```python
from build123d import *

# Parameters (mm, degrees)
BOSS_EXTRUDE1_DEPTH  = 8
M3_CLEARANCE_HOLE1_D = 3.6
FILLET1_R            = 1
SKETCH5_W            = 4
SKETCH5_H            = 7
CUT_EXTRUDE1_DEPTH   = 4
FILLET2_R            = 1


with BuildPart() as part:
    # Sketch1 → Boss-Extrude1 (new body)
    with BuildSketch(Plane.XY):
        Polygon((-16.25, -7.5), (-11.5, -7.5), (-11.5, 0), (3.5, 0), (3.5, 4), (11.5, 4), (11.5, -7.5), (16.25, -7.5), (16.25, 7), (-16.25, 7), align=None)
    extrude(amount=BOSS_EXTRUDE1_DEPTH)

    # M3 Clearance Hole1 (through all)
    with Locations(Plane(origin=(0, 7, 0), x_dir=(1, 0, 0), z_dir=(0, 1, 0))):
        with Locations((13.75, -4), (-13.75, -4)):
            Hole(M3_CLEARANCE_HOLE1_D / 2)

    # Fillet1
    fillet1_edges = [part.edges().sort_by_distance(p)[0] for p in [
        (-16.25, -0.25, 8),
        (-16.25, -0.25, 0),
        (16.25, -0.25, 0),
        (16.25, -0.25, 8),
    ]]
    fillet(fillet1_edges, radius=FILLET1_R)

    # Sketch5 → Cut-Extrude1 (cut)
    with BuildSketch(Plane(origin=(0, 0, 0), x_dir=(-1, 0, 0), z_dir=(0, 0, -1))):
        with Locations((-9, 3.5)):
            Rectangle(SKETCH5_W, SKETCH5_H)
    extrude(amount=-CUT_EXTRUDE1_DEPTH, mode=Mode.SUBTRACT)

    # Fillet2
    fillet2_edges = [part.edges().sort_by_distance(p)[0] for p in [
        (11, 5.5, 4),
        (7, 5.5, 4),
    ]]
    fillet(fillet2_edges, radius=FILLET2_R)


solid = part.part
```
Check sheet for the modelled part. Datum: model origin and axes. Units: mm. A direction names the side the tool comes from. Give positions to 0.01 mm unless a question says otherwise; leave off trailing zeros. Order: outer loops, then holes, each group sorted by start corner. A loop starts at its lowest first (then second) coordinate and runs counter-clockwise, first axis right, second up. Notation, with made-up numbers: (84, -31) -> (135, -31) arc R15 ccw to (135, -12) -> close; hole circle Ø4 at (55.5, -19.5). An arc over 180 degrees is marked (long way). Use CSV: the item, a comma, the result in double quotes. Start each with the question number.
1) Go/stop test with flat-tipped pins: P1, Ø1, axis at x = 8.5, y = 5, coming from the -Z side; P2, Ø1.5, axis at x = -1.5, z = 4, coming from the -Y side. Record where each tip stops, or that it passes through.
2) Set-up check for faces 1 (the face through (-4, 0, 4)), 2 (the face through (14, -7.5, 2)), 3 (the face through (11, 5, 1)): record each of +Z, -Z, +X, -X, +Y, -Y from which the full face is reachable in a straight line by a thin tool's end or side.
3) Mould release check, pull along X, two halves, no side actions. Record for faces 4 (the face through (7.285, 5.521, 3.699)), 5 (the face through (16.25, 0, 4)), 6 (the face through (13, 0, 0)): released by +X, released by -X, zero draft, split by the parting line, or undercut.
4) Sectioned sample at D-D, the plane x = 13. Record the boundary of the cut face in (y, z), plus the area to 3 significant figures.
5) Material ranges on line 1 (X direction, y = -0.25, z = 4); line 2 (X direction, y = 3.5, z = 4); line 3 (Z direction, x = -13.75, y = 2.5), recorded low to high. Write a range as from..to.
6) Sectioned sample at C-C, the plane y = -5.5. Record the boundary of the cut face in (x, z).
7) Sectioned sample at A-A, the plane y = 0.75. Record the boundary of the cut face in (x, z).
8) Sectioned sample at B-B, the plane x = -13.75. Record the boundary of the cut face in (y, z), plus the area to 3 significant figures.
Recorded:
1,P1,"z = 4"
1,P2,"y = 0"
2,face 1,"+Z, -Z, -Y"
2,face 2,"+Z, -Z, +X, -X, -Y"
2,face 3,"-Z, +Y, -Y"
3,face 4,"undercut"
3,face 5,"released by +X"
3,face 6,"zero draft"
4,outline,"(-7.5, 0) -> (7, 0) -> (7, 2.36) -> (-7.5, 2.36) -> close; (-7.5, 5.64) -> (7, 5.64) -> (7, 8) -> (-7.5, 8) -> close"
4,area,"68.5 mm2"
5,line 1,"-16.25..-15.55, -11.95..-11.5, 11.5..11.95, 15.55..16.25"
5,line 2,"-16.25..-15.55, -11.95..3.5, 11.5..11.95, 15.55..16.25"
5,line 3,"0..2.2, 5.8..8"
6,outline,"(-16.25, 1) arc R1 ccw to (-15.25, 0) -> (-11.5, 0) -> (-11.5, 8) -> (-15.25, 8) arc R1 ccw to (-16.25, 7) -> close; (11.5, 0) -> (15.25, 0) arc R1 ccw to (16.25, 1) -> (16.25, 7) arc R1 ccw to (15.25, 8) -> (11.5, 8) -> close; hole circle Ø3.6 at (-13.75, 4); hole circle Ø3.6 at (13.75, 4)"
7,outline,"(-16.25, 1) arc R1 ccw to (-15.25, 0) -> (3.5, 0) -> (3.5, 8) -> (-15.25, 8) arc R1 ccw to (-16.25, 7) -> close; (11.5, 0) -> (15.25, 0) arc R1 ccw to (16.25, 1) -> (16.25, 7) arc R1 ccw to (15.25, 8) -> (11.5, 8) -> close; hole circle Ø3.6 at (-13.75, 4); hole circle Ø3.6 at (13.75, 4)"
8,outline,"(-7.5, 0) -> (7, 0) -> (7, 2.2) -> (-7.5, 2.2) -> close; (-7.5, 5.8) -> (7, 5.8) -> (7, 8) -> (-7.5, 8) -> close"
8,area,"63.8 mm2"
